from build123d import *

# Parameters (mm, degrees)
SKETCH1_R            = 4.445
BOSS_EXTRUDE1_DEPTH  = 127
SKETCH7_W            = 6.35
SKETCH7_H            = 57.15
SKETCH7_H_2          = 80.01
SKETCH7_H_3          = 66.04
BOSS_EXTRUDE4_DEPTH  = 127
CUT_EXTRUDE2_REACH   = 191.917
SKETCH8_R            = 1.0999978
CUT_EXTRUDE4_REACH   = 200.726
SKETCH11_W           = 42.926
SKETCH11_H           = 101.345290086
FILLET1_R            = 17.78
CUT_EXTRUDE6_REACH   = 200.726
SKETCH14_R           = 1.249999967
SKETCH15_W           = 6.35
SKETCH15_H           = 127
CUT_EXTRUDE7_DEPTH   = 7.62
SKETCH16_W           = 12.827354957
SKETCH16_H           = 49.53
BOSS_EXTRUDE5_DEPTH  = 16.256
SKETCH17_W           = 38.227354957
SKETCH17_H           = 49.53
BOSS_EXTRUDE6_DEPTH  = 2.54
SKETCH18_W           = 21.632068301
SKETCH18_H           = 15.24
BOSS_EXTRUDE7_DEPTH  = 101.345290086
FILLET2_R            = 12.7
SKETCH23_R           = 0.95
CUT_EXTRUDE8_DEPTH   = 25.4
CHAMFER1_SIZE        = 2.54
CHAMFER1_SIZE2       = 5.447047578
BOSS_EXTRUDE10_DEPTH = 38.1
SKETCH26_W           = 73.406
SKETCH26_H           = 32.385
BOSS_EXTRUDE11_DEPTH = 12.827354957
FILLET3_R            = 12.7
BOSS_EXTRUDE12_DEPTH = 8.89
FILLET4_R            = 7.62
SKETCH28_W           = 6.35
SKETCH28_H           = 12.7
CUT_EXTRUDE9_DEPTH   = 25.4
SKETCH29_W           = 12.7
SKETCH29_H           = 6.35
CUT_EXTRUDE10_DEPTH  = 25.4


with BuildPart() as part:
    # Sketch1 → Boss-Extrude1 (new body)
    with BuildSketch(Plane.XY):
        with BuildLine():
            Line((0, -7.62), (127, -7.62))
            ThreePointArc((127, -7.62), (134.62, 0), (127, 7.62))
            Line((127, 7.62), (0, 7.62))
            ThreePointArc((0, 7.62), (-7.62, 0), (0, -7.62))
        make_face()
        with Locations((127, 0)):
            Circle(SKETCH1_R, mode=Mode.SUBTRACT)
        Circle(SKETCH1_R, mode=Mode.SUBTRACT)
    extrude(amount=BOSS_EXTRUDE1_DEPTH)

    # Sketch7 → Boss-Extrude4 (add)
    with BuildSketch(Plane.XY.offset(127)):
        with Locations((92.075, -36.195)):
            Rectangle(SKETCH7_W, SKETCH7_H)
        with Locations((12.319, 0)):
            Rectangle(SKETCH7_W, SKETCH7_H_2)
        with Locations((61.595, 31.75)):
            Rectangle(SKETCH7_W, SKETCH7_H_3)
    extrude(amount=-BOSS_EXTRUDE4_DEPTH)

    # Sketch8 → Cut-Extrude2 (cut, up to next)
    with BuildSketch(Plane.ZY.offset(-9.144), mode=Mode.PRIVATE) as cut_extrude2_sk1:
        with Locations(Location((104.763196308, 34.801440473, 0), (0, 0, 270))):
            Circle(SKETCH8_R)
    cut_extrude2_tool1 = extrude(cut_extrude2_sk1.sketch, amount=-CUT_EXTRUDE2_REACH, mode=Mode.PRIVATE) & part.part
    # Sketch8 → Cut-Extrude2 (cut, up to next)
    with BuildSketch(Plane.ZY.offset(-9.144), mode=Mode.PRIVATE) as cut_extrude2_sk2:
        with Locations(Location((104.763196308, -31.698559623, 0), (0, 0, 270))):
            Circle(SKETCH8_R)
    cut_extrude2_tool2 = extrude(cut_extrude2_sk2.sketch, amount=-CUT_EXTRUDE2_REACH, mode=Mode.PRIVATE) & part.part
    # Sketch8 → Cut-Extrude2 (cut, up to next)
    with BuildSketch(Plane.ZY.offset(-9.144), mode=Mode.PRIVATE) as cut_extrude2_sk3:
        with Locations(Location((20.763196414, -31.698559623, 0), (0, 0, 270))):
            Circle(SKETCH8_R)
    cut_extrude2_tool3 = extrude(cut_extrude2_sk3.sketch, amount=-CUT_EXTRUDE2_REACH, mode=Mode.PRIVATE) & part.part
    # Sketch8 → Cut-Extrude2 (cut, up to next)
    with BuildSketch(Plane.ZY.offset(-9.144), mode=Mode.PRIVATE) as cut_extrude2_sk4:
        with Locations(Location((20.763196414, 34.801440473, 0), (0, 0, 270))):
            Circle(SKETCH8_R)
    cut_extrude2_tool4 = extrude(cut_extrude2_sk4.sketch, amount=-CUT_EXTRUDE2_REACH, mode=Mode.PRIVATE) & part.part
    add(cut_extrude2_tool1.solids().sort_by_distance((9.144, 34.80144, 104.763196))[0], mode=Mode.SUBTRACT)
    add(cut_extrude2_tool2.solids().sort_by_distance((9.144, -31.69856, 104.763196))[0], mode=Mode.SUBTRACT)
    add(cut_extrude2_tool3.solids().sort_by_distance((9.144, -31.69856, 20.763196))[0], mode=Mode.SUBTRACT)
    add(cut_extrude2_tool4.solids().sort_by_distance((9.144, 34.80144, 20.763196))[0], mode=Mode.SUBTRACT)

    # Sketch11 → Cut-Extrude4 (cut, up to next)
    with BuildSketch(Plane.XZ.offset(7.62), mode=Mode.PRIVATE) as cut_extrude4_sk1:
        with Locations((36.957, 63.5)):
            Rectangle(SKETCH11_W, SKETCH11_H)
    cut_extrude4_tool1 = extrude(cut_extrude4_sk1.sketch, amount=-CUT_EXTRUDE4_REACH, mode=Mode.PRIVATE) & part.part
    add(cut_extrude4_tool1.solids().sort_by_distance((36.957, -7.62, 63.5))[0], mode=Mode.SUBTRACT)

    # Fillet1
    fillet1_edges = [part.edges().sort_by_distance(p)[0] for p in [
        (9.144, -7.62, 63.5),
        (9.144, 7.62, 63.5),
    ]]
    fillet(fillet1_edges, radius=FILLET1_R)

    # Sketch14 → Cut-Extrude6 (cut, up to next)
    with BuildSketch(Plane(origin=(0, 7.62, 0), x_dir=(1, 0, 0), z_dir=(0, 1, 0)), mode=Mode.PRIVATE) as cut_extrude6_sk1:
        with Locations(Location((119.866000044, -42.90656366, 0), (0, 0, 270))):
            Circle(SKETCH14_R)
    cut_extrude6_tool1 = extrude(cut_extrude6_sk1.sketch, amount=-CUT_EXTRUDE6_REACH, mode=Mode.PRIVATE) & part.part
    # Sketch14 → Cut-Extrude6 (cut, up to next)
    with BuildSketch(Plane(origin=(0, 7.62, 0), x_dir=(1, 0, 0), z_dir=(0, 1, 0)), mode=Mode.PRIVATE) as cut_extrude6_sk2:
        with Locations(Location((70.866, -42.90656366, 0), (0, 0, 270))):
            Circle(SKETCH14_R)
    cut_extrude6_tool2 = extrude(cut_extrude6_sk2.sketch, amount=-CUT_EXTRUDE6_REACH, mode=Mode.PRIVATE) & part.part
    # Sketch14 → Cut-Extrude6 (cut, up to next)
    with BuildSketch(Plane(origin=(0, 7.62, 0), x_dir=(1, 0, 0), z_dir=(0, 1, 0)), mode=Mode.PRIVATE) as cut_extrude6_sk3:
        with Locations(Location((70.866, -100.906563738, 0), (0, 0, 270))):
            Circle(SKETCH14_R)
    cut_extrude6_tool3 = extrude(cut_extrude6_sk3.sketch, amount=-CUT_EXTRUDE6_REACH, mode=Mode.PRIVATE) & part.part
    # Sketch14 → Cut-Extrude6 (cut, up to next)
    with BuildSketch(Plane(origin=(0, 7.62, 0), x_dir=(1, 0, 0), z_dir=(0, 1, 0)), mode=Mode.PRIVATE) as cut_extrude6_sk4:
        with Locations(Location((119.866000044, -100.906563738, 0), (0, 0, 270))):
            Circle(SKETCH14_R)
    cut_extrude6_tool4 = extrude(cut_extrude6_sk4.sketch, amount=-CUT_EXTRUDE6_REACH, mode=Mode.PRIVATE) & part.part
    add(cut_extrude6_tool1.solids().sort_by_distance((119.866, 7.62, 42.906564))[0], mode=Mode.SUBTRACT)
    add(cut_extrude6_tool2.solids().sort_by_distance((70.866, 7.62, 42.906564))[0], mode=Mode.SUBTRACT)
    add(cut_extrude6_tool3.solids().sort_by_distance((70.866, 7.62, 100.906564))[0], mode=Mode.SUBTRACT)
    add(cut_extrude6_tool4.solids().sort_by_distance((119.866, 7.62, 100.906564))[0], mode=Mode.SUBTRACT)

    # Sketch15 → Cut-Extrude7 (cut)
    with BuildSketch(Plane(origin=(0, 64.77, 0), x_dir=(1, 0, 0), z_dir=(0, 1, 0))):
        with Locations((61.595, -63.5)):
            Rectangle(SKETCH15_W, SKETCH15_H)
    extrude(amount=-CUT_EXTRUDE7_DEPTH, mode=Mode.SUBTRACT)

    # Sketch16 → Boss-Extrude5 (add)
    with BuildSketch(Plane.ZY.offset(-58.42)):
        with Locations((6.413677479, 32.385)):
            Rectangle(SKETCH16_W, SKETCH16_H)
    extrude(amount=BOSS_EXTRUDE5_DEPTH)

    # Sketch17 → Boss-Extrude6 (add)
    with BuildSketch(Plane.ZY.offset(-42.164)):
        with Locations((19.113677479, 32.385)):
            Rectangle(SKETCH17_W, SKETCH17_H)
    extrude(amount=BOSS_EXTRUDE6_DEPTH)

    # Sketch18 → Boss-Extrude7 (add)
    with BuildSketch(Plane.XY.offset(12.827354957)):
        with Locations((50.440034151, 0)):
            Rectangle(SKETCH18_W, SKETCH18_H)
    extrude(amount=BOSS_EXTRUDE7_DEPTH)

    # Fillet2
    fillet2_edges = [part.edges().sort_by_distance(p)[0] for p in [
        (15.494, 7.62, 6.413677479),
        (15.494, -7.62, 120.586322521),
        (15.494, 7.62, 120.586322521),
    ]]
    fillet(fillet2_edges, radius=FILLET2_R)

    # Sketch23 → Cut-Extrude8 (cut)
    with BuildSketch(Plane(origin=(95.25, 0, 0), x_dir=(0, 0, -1), z_dir=(1, 0, 0))):
        with Locations(Location((-105.41, -10.922, 0), (0, 0, 90))):
            Circle(SKETCH23_R)
        with Locations(Location((-22.81, -10.922, 0), (0, 0, 270))):
            Circle(SKETCH23_R)
        with Locations(Location((-22.81, -59.222, 0), (0, 0, 90))):
            Circle(SKETCH23_R)
        with Locations(Location((-105.41, -59.222, 0), (0, 0, 270))):
            Circle(SKETCH23_R)
    extrude(amount=-CUT_EXTRUDE8_DEPTH, mode=Mode.SUBTRACT)

    # Chamfer1
    chamfer1_edges = [part.edges().sort_by_distance(p)[0] for p in [
        (95.25, -64.77, 63.5),
    ]]
    chamfer1_side = [part.faces().sort_by_distance(p)[0] for p in [
        (95.25, -36.196757503, 63.499045346),
    ]]
    chamfer(chamfer1_edges, length=CHAMFER1_SIZE, length2=CHAMFER1_SIZE2, reference=chamfer1_side[0])

    # Sketch25 → Boss-Extrude10 (add)
    with BuildSketch(Plane.XY.offset(91.44)):
        Polygon((127, -7.62), (95.25, -7.62), (95.25, -62.23), align=None)
    extrude(amount=-BOSS_EXTRUDE10_DEPTH)

    # Sketch26 → Boss-Extrude11 (add)
    with BuildSketch(Plane(origin=(0, 0, 0), x_dir=(-1, 0, 0), z_dir=(0, 0, -1))):
        with Locations((-52.197, -23.8125)):
            Rectangle(SKETCH26_W, SKETCH26_H)
    extrude(amount=-BOSS_EXTRUDE11_DEPTH)

    # Fillet3
    fillet3_edges = [part.edges().sort_by_distance(p)[0] for p in [
        (88.9, -40.005, 6.413677479),
    ]]
    fillet(fillet3_edges, radius=FILLET3_R)

    # Sketch27 → Boss-Extrude12 (add)
    with BuildSketch(Plane(origin=(0, 0, 0), x_dir=(-1, 0, 0), z_dir=(0, 0, -1))):
        Polygon((-64.77, 7.62), (-64.77, 45.72), (-96.52, 7.62), align=None)
    extrude(amount=-BOSS_EXTRUDE12_DEPTH)

    # Fillet4
    fillet4_edges = [part.edges().sort_by_distance(p)[0] for p in [
        (96.52, 7.62, 4.445),
        (64.77, 45.72, 4.445),
    ]]
    fillet(fillet4_edges, radius=FILLET4_R)

    # Sketch28 → Cut-Extrude9 (cut)
    with BuildSketch(Plane.XZ.offset(7.62)):
        with Locations((52.681214832, 95.25)):
            Rectangle(SKETCH28_W, SKETCH28_H)
    extrude(amount=-CUT_EXTRUDE9_DEPTH, mode=Mode.SUBTRACT)

    # Sketch29 → Cut-Extrude10 (cut)
    with BuildSketch(Plane(origin=(64.77, 0, 0), x_dir=(0, 0, -1), z_dir=(1, 0, 0))):
        with Locations((-95.25, 36.195)):
            Rectangle(SKETCH29_W, SKETCH29_H)
    extrude(amount=-CUT_EXTRUDE10_DEPTH, mode=Mode.SUBTRACT)


solid = part.part
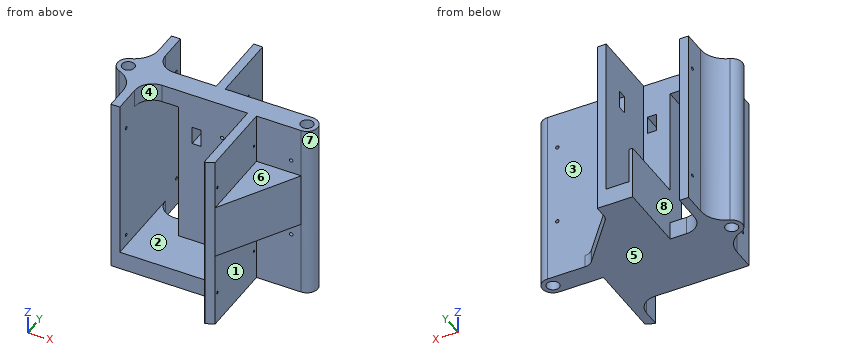
The listing builds one solid part. Answer for the finished solid, in the listing's coordinates (mm). Face numbers are marked on the shaded views. A direction names the side the tool comes from. Give positions to 0.01 mm unless a question says otherwise; leave off trailing zeros. Order: outer loops, then holes, each group sorted by start corner. A loop starts at its lowest first (then second) coordinate and runs counter-clockwise, first axis right, second up. Notation, with made-up numbers: (84, 52.5) - (129, 52.5) arc R10 cw to (129, 60.5) - close; hole circle Ø10 at (75, 5.25). An arc over 180 degrees is marked (long way). Answer as CSV lines item,"result".
Q1. Which of the six approach directions +Z, -Z, +X, -X, +Y, -Y give full straight-line access (tool end or side, diameter ignored) to the marked faces 1, 2, 3 and 4?
Answer key:
face 1,"-Z, +X, -Y"
face 2,"-Y"
face 3,"+Z, +X, +Y"
face 4,"+Z, -Y"
Q2. Straight lines are drawn through the part: L1, parallel to X at y = -31.5, z = 29; L2, parallel to Z at x = 119.5, y = 0; L3, parallel to Y at x = 127, z = 44 (3 decimals). For each, find the intervals that lie inside material, in ascending order.
Answer key:
L1,"x = 9.14 to 15.49, 88.9 to 95.25"
L2,"z = 0 to 41.71, 44.1 to 99.71, 102.1 to 127"
L3,"y = -7.62 to -4.445, 4.445 to 7.62"
Q3. A cutting plane is placed at A-A, the plane x = 34. Determine the outline of the cut face in (y, z) (3 decimals).
Answer key:
outline,"(-40.005, 0) - (7.62, 0) - (7.62, 12.827) - (-40.005, 12.827) - close; (-7.62, 114.173) - (7.62, 114.173) - (7.62, 127) - (-7.62, 127) - close"
Q4. Determine the mould class of the marked faces 5, 6, 7 and 8 for opening direction Z: pulls with the +Z half, pulls with the -Z half, needs draft (parallel to the pull), parting line crosses it, or undercut.
Answer key:
face 5,"pulls with the -Z half"
face 6,"pulls with the +Z half"
face 7,"needs draft"
face 8,"undercut"
Q5. Each of these flat-tipped pins is pushed along its axis until it touches: pin 1 Ø7 at (x, z) = (61.5, 97) entering from -Y; pin 2 Ø17.5 at (y, z) = (29.5, 70) entering from -X; pin 3 Ø1.5 at (x, z) = (10.5, 38.5) entering from +Y (3 decimals). Where does it stop, or does it pass through?
Answer key:
pin 1,"stops at y = -7.62"
pin 2,"stops at x = 8.87"
pin 3,"stops at y = 40.005"
Q6. A cutting plane is placed at B-B, the plane y = 0. Count the separate pieces of the cut face and the enclosed holes in it, and give its area (3 significant figures).
Answer key:
separate pieces,"3"
enclosed holes,"6"
area,"13,300 mm^2"
